Check sheet for the modelled part. Datum: model origin and axes. Units: mm. Face numbers are marked on the shaded views. A direction names the side the tool comes from. Round coordinates to 2 decimals unless told otherwise and drop trailing zeros. Order: outer loops, then holes, each group sorted by start corner. A loop starts at its lowest first (then second) coordinate and runs counter-clockwise, first axis right, second up.
Autodesk Inventor part; units mm, degrees
ref_plane "YZ Plane" through (0, 0, 0) normal (1, 0, 0) x (0, 1, 0)
ref_plane "XZ Plane" through (0, 0, 0) normal (0, 1, 0) x (-1, 0, 0)
ref_plane "XY Plane" through (0, 0, 0) normal (0, 0, 1) x (1, 0, 0)
sketch "Esboço1" plane through (0, 0, 0) normal (0, 0, 1) x (1, 0, 0)
  line L0 (-7.2, 0) -> (1.2, 0) construction
  line L1 (0, -13.5) -> (0, 42.5) construction
  line L2 (0, 34.5) -> (0, -5.5)
  line L3 (0, -5.5) -> (-2, -5.5)
  line L4 (-2, -5.5) -> (-2, 0)
  line L5 (-2, 0) -> (-6, 0)
  line L6 (-6, 0) -> (-6, 1.5)
  line L7 (-6, 1.5) -> (-5, 1.5)
  line L8 (-5, 1.5) -> (-5, 34.5)
  line L9 (-5, 34.5) -> (0, 34.5)
  point P0 (0, 0)
  dimension "d0" = 10
  dimension "d1" = 12
  dimension "d2" = 1.5
  dimension "d3" = 5.5
  dimension "d4" = 33
  dimension "d7" = 4
  dimension "d21" = 40
revolve "Revolução1" add sketch "Esboço1" angle 360 about axis through (0, -10, 0) along (0, 1, 0)
sketch "Esboço2" plane through (0, 34.5, 0) normal (0, 1, 0) x (1, 0, 0)
  circle A0 centre (0, 0) radius 5
hole "Furo1" at (0, 34.5, 0) direction (0, -1, 0) diameter 4.917 depth 15 tip angle 118
thread "Rosca1"
chamfer "Chanfro1" distance 0.3 angle 45 3 edges at (2, -5.5, 0) (5, 34.5, 0) (0, 34.5, -2.4585)
properties part number "Compensador Haste" material "Aço SAE 1045"
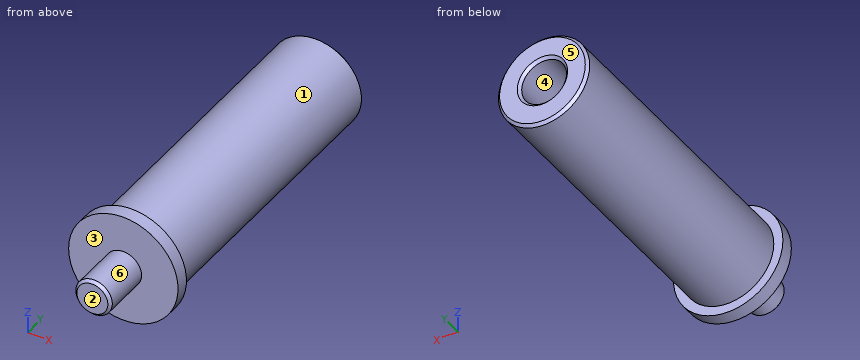
Item 1: Go/stop test with flat-tipped pins: P1, Ø6, axis at y = 29.5, z = 0.5, coming from the +X side; P2, Ø1, axis at x = -2, z = -4.5, coming from the -Y side; P3, Ø4, axis at y = 26.5, z = -3.5, coming from the +X side. Record where each tip stops, or that it passes through.
Answer:
P1: stops at x = 5
P2: stops at y = 0
P3: stops at x = 4.77
Item 2: Access from +Z, -Z, +X, -X, +Y, -Y to the whole of each face (thin tool, end or side, straight path). Record for the marked faces 1, 2 and 3.
Answer:
face 1: +Y
face 2: +Z, -Z, +X, -X, -Y
face 3: -Y
Item 3: Sectioned sample at C-C (y = -1). Record the cut outline in (x, z).
Answer:
outline: circle Ø4 at (0, 0)
Item 4: Release check for a two-part mould opening along Z. For the marked faces 4, 5 and 6 record: released by +Z, released by -Z, zero draft, split by the parting line, or undercut.
Answer:
face 4: undercut
face 5: zero draft
face 6: split by the parting line
Item 5: Scan lines: line 1 along Z through (x, y) = (0, 25.5); line 2 along Y through (x, z) = (3.25, 0.5); line 3 along X through (y, z) = (28.5, 2). Record each from-to range of solid material in increasing order.
Answer:
line 1: z = -5 to -2.46, 2.46 to 5
line 2: y = 0 to 34.5
line 3: x = -4.58 to -1.43, 1.43 to 4.58
Item 6: Sectioned sample at B-B (y = 15). Record the cut outline in (x, z), and give its area (3 significant figures).
Answer:
outline: circle Ø10 at (0, 0)
area: 78.5 mm2
Item 7: Sectioned sample at A-A (y = 32.5). Record the cut outline in (x, z), and give its area (3 significant figures).
Answer:
outline: circle Ø10 at (0, 0); hole circle Ø4.92 at (0, 0)
area: 59.6 mm2
